Geometry: see drawing. Coordinates: mm, zero at the bounding-box minimum. A direction names the side the tool comes from. Coordinates: 2 decimals unless noted, no trailing zeros. Loops run counter-clockwise (first coordinate to the right, second up) from the corner with the lowest first, then second, coordinate; pieces in that order, holes last. Notation, with made-up numbers: (5, 67) - (64, 67) arc R13 ccw to (64, 77) - close; hole circle Ø5 at (87.5, 85.25). An arc over 180 degrees is marked (long way). Use a Markdown table: item, result. Add a question column.
1. Section query A-A on x = 7.75. Return the cut outline in (y, z), then the cut area to 4 significant figures.
2. Section query D-D on y = 56. Return the cut outline in (x, z), then the cut area to 3 significant figures.
3. Section query C-C on y = 15.5. Return the cut outline in (x, z).
4. Access query for the marked faces 1, 2 and 3. Directions: +Z, -Z, +X, -X, +Y, -Y. A direction counts if a zero-diameter tool reaches every point of the face in a straight line with its end or side. Return the directions, or none.
5. Ray query, L1, parallel to Y at x = 0.6, z = 7.75; L2, parallel to Z at x = 0.7, y = 45.5; L3, parallel to Y at x = 12, z = 4.75. Return the intervals inside material, ascending. Write a range as [from, to].
6. Contact query for flat-ended pins moving along their axis: P1, Ø1.5, axis at y = 13.5, z = 3.5, coming from the +X side; P2, Ø5, axis at y = 7.5, z = 12.5, coming from the -X side; P3, Ø6, axis at y = 6, z = 5.5, coming from the -X side; P4, Ø8, axis at y = 15, z = 7, coming from the +X side. Output: stop coordinate, or through.
7. Section query B-B on z = 13. Return the cut outline in (x, y).
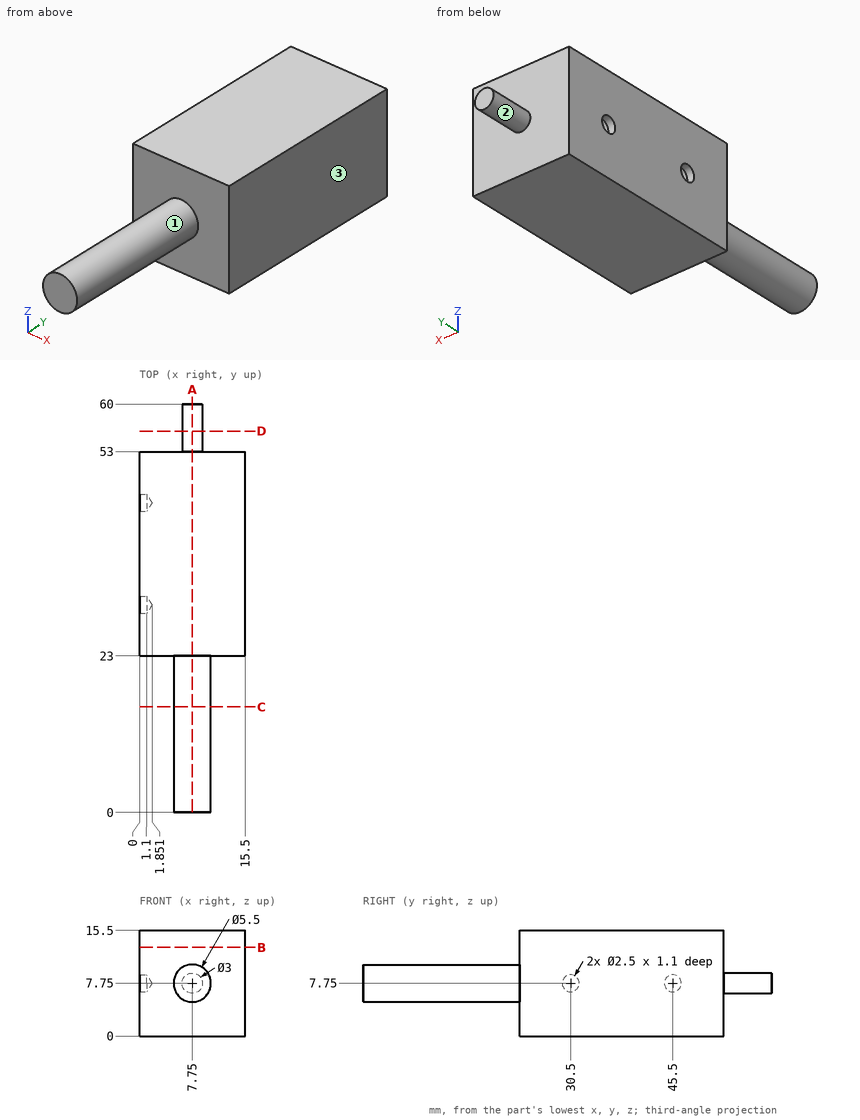
Resolved:
| question | item | result |
|---|---|---|
| 1 | outline | (0, 5) - (23, 5) - (23, 0) - (53, 0) - (53, 6.25) - (60, 6.25) - (60, 9.25) - (53, 9.25) - (53, 15.5) - (23, 15.5) - (23, 10.5) - (0, 10.5) - close |
| 1 | area | 612.5 mm² |
| 2 | outline | circle Ø3 at (7.75, 7.75) |
| 2 | area | 7.07 mm² |
| 3 | outline | circle Ø5.5 at (7.75, 7.75) |
| 4 | face 1 | -Y |
| 4 | face 2 | +Y |
| 4 | face 3 | +Z, -Z, +X, +Y, -Y |
| 5 | L1 | [23, 29.25], [31.75, 44.25], [46.75, 53] |
| 5 | L2 | [0, 6.5], [9, 15.5] |
| 5 | L3 | [23, 53] |
| 6 | P1 | through |
| 6 | P2 | x = 6.17 |
| 6 | P3 | x = 5 |
| 6 | P4 | x = 10.5 |
| 7 | outline | (0, 23) - (15.5, 23) - (15.5, 53) - (0, 53) - close |
